```python
from build123d import *

# Parameters (mm, degrees)
SKETCH1_R           = 1.5
BOSS_EXTRUDE1_DEPTH = 7
BOSS_EXTRUDE2_DEPTH = 3


with BuildPart() as part:
    # Sketch1 → Boss-Extrude1 (new body)
    with BuildSketch(Plane.XY):
        with Locations((-63.49476159, 14.978708134)):
            Circle(SKETCH1_R)
    extrude(amount=BOSS_EXTRUDE1_DEPTH)

    # Sketch2 → Boss-Extrude2 (add)
    with BuildSketch(Plane(origin=(0, 0, 0), x_dir=(-1, 0, 0), z_dir=(0, 0, -1))):
        Polygon((63.49476159, 12.091956788), (65.99476159, 13.535332461), (65.99476159, 16.422083807), (63.49476159, 17.86545948), (60.99476159, 16.422083807), (60.99476159, 13.535332461), align=None)
    extrude(amount=BOSS_EXTRUDE2_DEPTH)


solid = part.part
```
Geometry: final body of the model. Coordinates: model frame, mm. A direction names the side the tool comes from. Coordinates: 2 decimals unless noted, no trailing zeros. Order: outer loops, then holes, each group sorted by start corner. A loop starts at its lowest first (then second) coordinate and runs counter-clockwise, first axis right, second up.
Item 1: Section query C-C (x = -62.55). Output: boundary loops of the cut face in (y, z), then the cut area to 3 significant figures.
Answer:
outline: (12.64, -3) - (17.32, -3) - (17.32, 0) - (16.14, 0) - (16.14, 7) - (13.81, 7) - (13.81, 0) - (12.64, 0) - close
area: 30.4 mm2
Item 2: Contact query for flat-ended pins moving along their axis: P1, Ø3, axis at y = 15, z = 2, coming from the +X side; P2, Ø1, axis at x = -63, z = 2.5, coming from the -Y side. Output: stop coordinate, or through.
Answer:
P1: stops at x = -61.99
P2: stops at y = 13.48
Item 3: Section query B-B (y = 15.35). Output: boundary loops of the cut face in (x, z).
Answer:
outline: (-65.99, -3) - (-60.99, -3) - (-60.99, 0) - (-62.04, 0) - (-62.04, 7) - (-64.95, 7) - (-64.95, 0) - (-65.99, 0) - close
Item 4: Material intervals for line 1 along Z through (x, y) = (-61.45, 13.6); line 2 along Y through (x, z) = (-63.45, 3); line 3 along X through (y, z) = (15.35, 4.75), sorted ascending.
Answer:
line 1: z = -3 to 0
line 2: y = 13.48 to 16.48
line 3: x = -64.95 to -62.04
Item 5: Access query for faces 1 (the face through (-62.688, 16.244, 3.451)), 2 (the face through (-62.23, 12.82, -1.48)). Directions: +Z, -Z, +X, -X, +Y, -Y. A direction counts if a zero-diameter tool reaches every point of the face in a straight line with its end or side. Return the directions, or none.
Answer:
face 1: +Z
face 2: +Z, -Z, +X, -Y
Item 6: Section query A-A (z = -1). Output: boundary loops of the cut face in (x, y), then the cut area to 3 significant figures.
Answer:
outline: (-65.99, 13.54) - (-63.49, 12.09) - (-60.99, 13.54) - (-60.99, 16.42) - (-63.49, 17.87) - (-65.99, 16.42) - close
area: 21.7 mm2
Item 7: Section query D-D (z = 1). Output: boundary loops of the cut face in (x, y).
Answer:
outline: circle Ø3 at (-63.49, 14.98)
